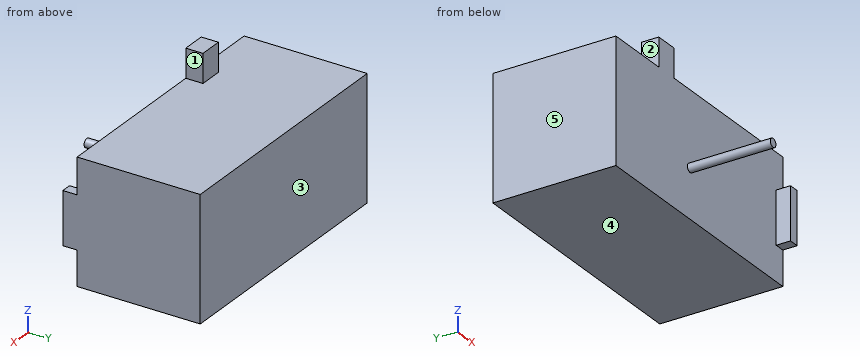
```python
from build123d import *

# Parameters (mm, degrees)
SKETCH_1_W      = 43
SKETCH_1_H      = 43
EXTRUDE_1_DEPTH = 90
SKETCH_2_R      = 1.5
EXTRUDE_2_DEPTH = 29
SKETCH_3_W      = 3.599409295
SKETCH_3_H      = 18.326935395
EXTRUDE_3_DEPTH = 5
SKETCH_4_W      = 8.291811564
SKETCH_4_H      = 6.001856053
EXTRUDE_4_DEPTH = 10


with BuildPart() as part:
    # 草图1 → 凸台-拉伸1 (new body)
    with BuildSketch(Plane(origin=(0, 0, 0), x_dir=(0, 0, -1), z_dir=(1, 0, 0))):
        with Locations((-21.5, 21.5)):
            Rectangle(SKETCH_1_W, SKETCH_1_H)
    extrude(amount=EXTRUDE_1_DEPTH)

    # 草图2 → 凸台-拉伸2 (add)
    with BuildSketch(Plane.XZ):
        with Locations(Location((40, 17, 0), (0, 0, 90))):
            Circle(SKETCH_2_R)
    extrude(amount=EXTRUDE_2_DEPTH)

    # 草图3 → 凸台-拉伸3 (add)
    with BuildSketch(Plane.XZ):
        with Locations((88.200295353, 21.266426497)):
            Rectangle(SKETCH_3_W, SKETCH_3_H)
    extrude(amount=EXTRUDE_3_DEPTH)

    # 草图4 → 凸台-拉伸4 (add)
    with BuildSketch(Plane.XY.offset(43)):
        with Locations((27.274280527, 3.000928027)):
            Rectangle(SKETCH_4_W, SKETCH_4_H)
    extrude(amount=EXTRUDE_4_DEPTH)


solid = part.part
```
Could you check a few things on this model? Use its own coordinates, in mm. Face numbers are marked on the shaded views. A direction names the side the tool comes from. Coordinates: 2 decimals unless noted, no trailing zeros. Write each loop counter-clockwise with the first axis right and the second up, starting at its lowest first coordinate (ties: lowest second). Pieces come first, ordered by that corner, then holes. Notation, with made-up numbers: M 41,20.5 L 79,20.5 A22 cw 79,48.5 Z; hole C 3.5,68 d10. An arc over 180 degrees is marked long. Answer as CSV lines item,"result". Start each with the question number.
1) I want a section at C-C, the plane y = 19. Please give me the cut outline in (x, z), and give its area (3 significant figures).
2) I want a section at B-B, the plane x = 40. Please give me the cut outline in (y, z).
3) We'd pull the mould along Z, two halves only. Please class the marked faces 4 and 5: +Z half, -Z half, draft (parallel to the pull), parting line (faces both ways), or undercut.
4) For the marked faces 1, 2 and 3, which set-ups out of +Z, -Z, +X, -X, +Y, -Y let a thin tool reach every point of the face, with its end or its side?
5) I want a section at A-A, the plane z = 17. Please give me the cut outline in (x, y), and give its area (4 significant figures).
6) Please list where this line runs through material, in increasing order: line 1 (Z direction, x = 74, y = 15.5). Write a range as from..to.
7) For P1, Ø4, axis at y = -2.5, z = 25, coming from the -X side; P2, Ø4, axis at x = 88, z = 22.5, coming from the -Y side; P3, Ø6, axis at x = 81, z = 45, coming from the -Y side; P4, Ø2, axis at y = -5.5, z = 25, coming from the +X side, each with a flat end and sliding along its axis, tell me the tip position at first contact or that it passes through.
Data:
1,outline,"M 0,0 L 90,0 L 90,43 L 0,43 Z"
1,area,"3,870 mm^2"
2,outline,"M -29,15.5 L 0,15.5 L 0,0 L 43,0 L 43,43 L 0,43 L 0,18.5 L -29,18.5 Z"
3,face 4,"-Z half"
3,face 5,"draft"
4,face 1,"+Z, +X, +Y, -Y"
4,face 2,"+Z, -X, +Y, -Y"
4,face 3,"+Z, -Z, +X, -X, +Y"
5,outline,"M 0,0 L 38.5,0 L 38.5,-29 L 41.5,-29 L 41.5,0 L 86.4,0 L 86.4,-5 L 90,-5 L 90,43 L 0,43 Z"
5,area,"3,975 mm^2"
6,line 1,"z = 0..43"
7,P1,"stops at x = 86.4"
7,P2,"stops at y = -5"
7,P3,"stops at y = 0"
7,P4,"stops at x = 90"
